```python
from build123d import *

# Parameters (mm, degrees)
SKETCH1_W          = 19.685
SKETCH1_H          = 40.64
EXTRUDE1_DEPTH     = 35.7632
CHAMFER1_SIZE      = 1.778
CHAMFER1_SIZE2     = 0.313509372
CHAMFER2_SIZE      = 1.778
CHAMFER2_SIZE2     = 0.313509372
CHAMFER3_SIZE      = 16.51
CHAMFER3_SIZE2     = 2.570638016
EXTRUDE2_REACH     = 44.294
SKETCH2_W          = 17.907
SKETCH2_H          = 14.732
CHAMFER4_SIZE      = 3.302
CHAMFER4_SIZE_2    = 2.312085291
SKETCH3_R          = 7.1755
EXTRUDE3_DEPTH     = 1.6256
CHAMFER5_SIZE      = 2.54
CHAMFER5_SIZE2     = 0.800858924
CHAMFER6_SIZE2     = 2.0955
CHAMFER6_SIZE      = 1.6256
SKETCH4_R          = 2.9591
CUT_EXTRUDE1_DEPTH = 10
SKETCH5_W          = 17.78
SKETCH5_H          = 2.413
EXTRUDE4_DEPTH     = 7.3152
CUT_EXTRUDE2_REACH = 43.041
SKETCH8_W          = 1.905
SKETCH8_H          = 3.81
EXTRUDE5_DEPTH     = 0.8636


# Some blends are built 0.0001 mm under size
with BuildPart() as part:
    # Sketch1 → Extrude1 (new body)
    with BuildSketch(Plane.XY):
        Rectangle(SKETCH1_W, SKETCH1_H)
    extrude(amount=EXTRUDE1_DEPTH)

    # Chamfer1
    chamfer1_edges = [part.edges().sort_by_distance(p)[0] for p in [
        (9.8425, 0, 35.7632),
    ]]
    chamfer1_side = [part.faces().sort_by_distance(p)[0] for p in [
        (9.8425, 0, 17.8816),
    ]]
    chamfer(chamfer1_edges, length=CHAMFER1_SIZE, length2=CHAMFER1_SIZE2, reference=chamfer1_side[0])

    # Chamfer2
    chamfer2_edges = [part.edges().sort_by_distance(p)[0] for p in [
        (-9.8425, 0, 35.7632),
    ]]
    chamfer2_side = [part.faces().sort_by_distance(p)[0] for p in [
        (-9.8425, 0, 17.8816),
    ]]
    chamfer(chamfer2_edges, length=CHAMFER2_SIZE, length2=CHAMFER2_SIZE2, reference=chamfer2_side[0])

    # Chamfer3
    chamfer3_edges = [part.edges().sort_by_distance(p)[0] for p in [
        (0, -20.32, 0),
    ]]
    chamfer3_side = [part.faces().sort_by_distance(p)[0] for p in [
        (0, 0, 0),
    ]]
    chamfer(chamfer3_edges, length=CHAMFER3_SIZE, length2=CHAMFER3_SIZE2, reference=chamfer3_side[0])

    # Sketch2 → Extrude2 (add, up to next)
    with BuildSketch(Plane(origin=(0, 0, 0), x_dir=(-1, 0, 0), z_dir=(0, 0, -1)), mode=Mode.PRIVATE) as extrude2_sk1:
        with Locations((0, -9.906)):
            Rectangle(SKETCH2_W, SKETCH2_H)
    extrude2_tool1 = extrude(extrude2_sk1.sketch, amount=-EXTRUDE2_REACH, mode=Mode.PRIVATE) - part.part
    add(extrude2_tool1.solids().sort_by_distance((0, -9.906, 0))[0])

    # Chamfer4
    # the kernel refuses this chamfer: 3.302, 2.312085291 mm, written as the material it takes off along each edge
    with BuildSketch(Plane(origin=(-17.481087464, -17.272, 0), x_dir=(0, 0.99975333476413, -0.022209674198457065), z_dir=(1, 0, 0))) as chamfer4_piece_1_section:
        Polygon((CHAMFER4_SIZE * 0.999753334764, CHAMFER4_SIZE * 0.0222096741985), (-CHAMFER4_SIZE_2 * 0.0222096742001, CHAMFER4_SIZE_2 * 0.999753334837), (0, 0), align=None)
    chamfer4_piece_1 = extrude(amount=34.962174929, mode=Mode.PRIVATE)
    chamfer4_piece_1 = split(chamfer4_piece_1, bisect_by=Plane(origin=(0, -15.96847592, 1.893097542), z_dir=(0, -0.15384816987279037, -0.9880944998464434)), keep=Keep.TOP, mode=Mode.PRIVATE)
    add(chamfer4_piece_1, mode=Mode.SUBTRACT)

    # Sketch3 → Extrude3 (add)
    with BuildSketch(Plane(origin=(0, 0, 0), x_dir=(-1, 0, 0), z_dir=(0, 0, -1))):
        with Locations(Location((0, 9.4615, 0), (0, 0, 180))):
            Circle(SKETCH3_R)
    extrude(amount=EXTRUDE3_DEPTH)

    # Chamfer5
    chamfer5_edges = [part.edges().sort_by_distance(p)[0] for p in [
        (0, 20.32, 0),
    ]]
    chamfer5_side = [part.faces().sort_by_distance(p)[0] for p in [
        (0, 20.32, 17.867899933),
    ]]
    chamfer(chamfer5_edges, length=CHAMFER5_SIZE, length2=CHAMFER5_SIZE2, reference=chamfer5_side[0])

    # Chamfer6
    chamfer6_edges = [part.edges().sort_by_distance(p)[0] for p in [
        (-7.1755, 9.4615, -1.6256),
    ]]
    chamfer6_side = [part.faces().sort_by_distance(p)[0] for p in [
        (-7.1755, 9.4615, -1.593088),
    ]]
    chamfer(chamfer6_edges, length=CHAMFER6_SIZE - 0.0001, length2=CHAMFER6_SIZE2 - 0.0001, reference=chamfer6_side[0])  # a hair under: the kernel refuses the full size

    # Sketch4 → Cut-Extrude1 (cut)
    with BuildSketch(Plane(origin=(0, 0, -1.6256), x_dir=(-1, 0, 0), z_dir=(0, 0, -1))):
        with Locations((0, 9.4615)):
            Circle(SKETCH4_R)
    extrude(amount=-CUT_EXTRUDE1_DEPTH, mode=Mode.SUBTRACT)

    # Sketch5 → Extrude4 (add)
    with BuildSketch(Plane(origin=(0, 20.32, 0), x_dir=(1, 0, 0), z_dir=(0, 1, 0))):
        with Locations((0, -8.2677)):
            Rectangle(SKETCH5_W, SKETCH5_H)
    extrude4 = extrude(amount=EXTRUDE4_DEPTH)

    # Sketch6 → Cut-Extrude2 (cut, up to next)
    with BuildSketch(Plane(origin=(0, 0, 7.0612), x_dir=(-1, 0, 0), z_dir=(0, 0, -1)), mode=Mode.PRIVATE) as cut_extrude2_sk1:
        with BuildLine():
            Line((-6.1849, 27.6352), (-3.7465, 27.6352))
            Line((-3.7465, 27.6352), (-3.7465, 26.996445941))
            ThreePointArc((-3.7465, 26.996445941), (-4.9657, 22.86), (-6.1849, 26.996445941))
            Line((-6.1849, 26.996445941), (-6.1849, 27.6352))
        make_face()
    cut_extrude2_tool1 = extrude(cut_extrude2_sk1.sketch, amount=-CUT_EXTRUDE2_REACH, mode=Mode.PRIVATE) & part.part
    # Sketch6 → Cut-Extrude2 (cut, up to next)
    with BuildSketch(Plane(origin=(0, 0, 7.0612), x_dir=(-1, 0, 0), z_dir=(0, 0, -1)), mode=Mode.PRIVATE) as cut_extrude2_sk2:
        with BuildLine():
            Line((3.7465, 27.6352), (6.1849, 27.6352))
            Line((6.1849, 27.6352), (6.1849, 26.996445941))
            ThreePointArc((6.1849, 26.996445941), (4.9657, 22.86), (3.7465, 26.996445941))
            Line((3.7465, 26.996445941), (3.7465, 27.6352))
        make_face()
    cut_extrude2_tool2 = extrude(cut_extrude2_sk2.sketch, amount=-CUT_EXTRUDE2_REACH, mode=Mode.PRIVATE) & part.part
    cut_extrude2_1 = cut_extrude2_tool1.solids().sort_by_distance((4.9657, 25.240383, 7.0612))[0]
    add(cut_extrude2_1, mode=Mode.SUBTRACT)
    cut_extrude2_2 = cut_extrude2_tool2.solids().sort_by_distance((-4.9657, 25.240383, 7.0612))[0]
    add(cut_extrude2_2, mode=Mode.SUBTRACT)
    cut_extrude2 = cut_extrude2_1 + cut_extrude2_2  # Cut-Extrude2 as one shape, for the pattern or mirror that repeats it

    # Sketch8 → Extrude5 (add)
    with BuildSketch(Plane(origin=(0, 0, 7.0612), x_dir=(-1, 0, 0), z_dir=(0, 0, -1))):
        with Locations((0, 22.225)):
            Rectangle(SKETCH8_W, SKETCH8_H)
    extrude5 = extrude(amount=EXTRUDE5_DEPTH)

    # Mirror1: Extrude4, Cut-Extrude2, Extrude5 across plane
    add(extrude4.mirror(Plane.ZX))
    add(cut_extrude2.mirror(Plane.ZX), mode=Mode.SUBTRACT)
    add(extrude5.mirror(Plane.ZX))


solid = part.part
```
The listing builds one solid part. Answer for the finished solid, in the listing's coordinates (mm). A direction names the side the tool comes from. Round coordinates to 2 decimals unless told otherwise and drop trailing zeros. Loops run counter-clockwise (first coordinate to the right, second up) from the corner with the lowest first, then second, coordinate; pieces in that order, holes last. Notation, with made-up numbers: (-6.75, 7) - (4.25, 7) arc R21 cw to (4.25, 24) - close; hole circle Ø9 at (82, 40.5). An arc over 180 degrees is marked (long way). Return JSON: item names as keys, results as strings. Group by question number.
1. Which of the six approach directions +Z, -Z, +X, -X, +Y, -Y give full straight-line access (tool end or side, diameter ignored) to faces 4 (the flat face through (-8.954, -12, 1)), 5 (the flat face through (0, 22, 6.198)), 6 (the flat face through (0, -23, 9.474)), 7 (the flat face through (8.954, -12, 1))?
2. The part is cut by section B-B on y = -0.5. Determine the outline of the cut face in (x, z), then the cut area to 3 significant figures.
3. Each of these flat-tipped pins is pushed along its axis until it touches: P1, Ø4, axis at x = -3.5, y = -15.5, coming from the -Z side; P2, Ø5, axis at x = 1, z = 32, coming from the -Y side; P3, Ø1.5, axis at x = -0.5, y = 22, coming from the -Z side. Where does it stop, or does it pass through?
4. The part is cut by section D-D on y = -21.5. Determine the outline of the cut face in (x, z), then the cut area to 3 significant figures.
5. Consider probe 1 along Y at (x, z) = (0, 6.5); probe 2 along Z at (x, y) = (-8.5, 15); probe 3 along Y at (x, z) = (-5, 23). Determine where each line is inside the solid, lowest interval first.
6. The mould has two halves that part along X. Classify faces 1 (the cylindrical face through (-5.05, -22.86, 8.25)), 2 (the flat face through (8.89, -24, 8)), 3 (the flat face through (8, -27.635, 8)): pulls with the +X half, pulls with the -X half, needs draft (parallel to the pull), parting line crosses it, or undercut.
7. The part is cut by section C-C on z = 11.5. Determine the outline of the cut face in (x, y), then the cut area to 3 significant figures.
Resolved:
{
 "1": {"face 4": "-Z, -X, -Y", "face 5": "-Z, +X, -X, +Y", "face 6": "+Z, +X, -X, -Y", "face 7": "-Z, +X, -Y"},
 "2": {"outline": "(-9.84, 0) - (9.84, 0) - (9.84, 33.99) - (9.53, 35.76) - (-9.53, 35.76) - (-9.84, 33.99) - close", "area": "703 mm²"},
 "3": {"P1": "stops at z = 0", "P2": "stops at y = -20.32", "P3": "stops at z = 6.2"},
 "4": {"outline": "(-8.89, 7.06) - (-0.95, 7.06) - (-0.95, 6.2) - (0.95, 6.2) - (0.95, 7.06) - (8.89, 7.06) - (8.89, 9.47) - (-8.89, 9.47) - close", "area": "44.5 mm²"},
 "5": {"probe 1": "y = -24.13 to 6.5, 12.42 to 24.13", "probe 2": "z = 0 to 35.76", "probe 3": "y = -20.32 to 20.32"},
 "6": {"face 1": "undercut", "face 2": "pulls with the +X half", "face 3": "needs draft"},
 "7": {"outline": "(-9.84, -20.32) - (9.84, -20.32) - (9.84, 20.32) - (-9.84, 20.32) - close", "area": "800 mm²"}
}
